from build123d import *

# Parameters (mm, degrees)
SKETCH1_W                     = 30
SKETCH1_H                     = 13.6
MAIN_SHAPE_DEPTH              = 6.35
SHOULDER_X_MOUNT_HOLES_D      = 1.9939
SHOULDER_X_MOUNT_HOLES_DEPTH  = 7.67
SHOULDER_X_MOUNT_HOLES_TIP    = 0.599027994
ELBOW_SERVO_MOUNT_HOLES_D     = 1.9939
ELBOW_SERVO_MOUNT_HOLES_DEPTH = 7.67
ELBOW_SERVO_MOUNT_HOLES_TIP   = 0.599027994
FILLET2_R                     = 3
WEIGHT_REMOVAL_DEPTH          = 7.35


with BuildPart() as part:
    # Sketch1 → main shape (new body)
    with BuildSketch(Plane.XY):
        Polygon((0, 0), (120, 0), (120, 30), (0, 30), (0, 17.159), (30, 17.159), (30, 12.841), (0, 12.841), align=None)
        with Locations((99, 15)):
            Rectangle(SKETCH1_W, SKETCH1_H, mode=Mode.SUBTRACT)
    extrude(amount=MAIN_SHAPE_DEPTH)

    # shoulder X mount holes
    with Locations(Plane.XY.offset(6.35)):
        with Locations((26.625, 26.625), (26.625, 3.375), (3.375, 3.375), (3.375, 26.625)):
            Hole(SHOULDER_X_MOUNT_HOLES_D / 2, depth=SHOULDER_X_MOUNT_HOLES_DEPTH)
            with Locations((0, 0, -(SHOULDER_X_MOUNT_HOLES_DEPTH + SHOULDER_X_MOUNT_HOLES_TIP / 2))):  # 118° drill point
                Cone(0, SHOULDER_X_MOUNT_HOLES_D / 2, SHOULDER_X_MOUNT_HOLES_TIP, mode=Mode.SUBTRACT)

    # elbow servo mount holes
    with Locations(Plane.XY.offset(6.35)):
        with Locations((81.5, 15), (116.5, 15)):
            Hole(ELBOW_SERVO_MOUNT_HOLES_D / 2, depth=ELBOW_SERVO_MOUNT_HOLES_DEPTH)
            with Locations((0, 0, -(ELBOW_SERVO_MOUNT_HOLES_DEPTH + ELBOW_SERVO_MOUNT_HOLES_TIP / 2))):  # 118° drill point
                Cone(0, ELBOW_SERVO_MOUNT_HOLES_D / 2, ELBOW_SERVO_MOUNT_HOLES_TIP, mode=Mode.SUBTRACT)

    # Fillet2
    fillet2_edges = [part.edges().sort_by_distance(p)[0] for p in [
        (0, 30, 3.175),
        (120, 30, 3.175),
        (120, 0, 3.175),
        (0, 0, 3.175),
    ]]
    fillet(fillet2_edges, radius=FILLET2_R)

    # Sketch8 → weight removal (cut, through all)
    with BuildSketch(Plane.XY):
        Polygon((36.41522176, 26), (55.5, 16.669663972), (74.58477824, 26), align=None)
        Polygon((36.41522176, 4), (74.58477824, 4), (55.5, 13.330336028), align=None)
        Polygon((78, 24.330336028), (78, 5.669663972), (58.91522176, 15), align=None)
        Polygon((33, 24.330336028), (52.08477824, 15), (33, 5.669663972), align=None)
    extrude(amount=WEIGHT_REMOVAL_DEPTH, mode=Mode.SUBTRACT)


solid = part.part
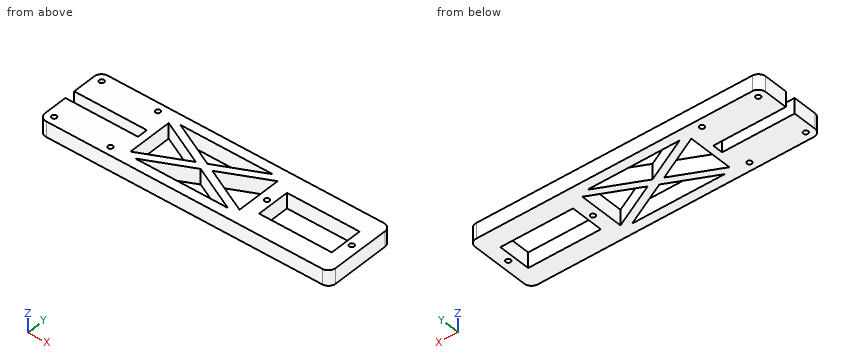
Could you check a few things on this model? Use its own coordinates, in mm. Give positions to 0.01 mm unless a question says otherwise; leave off trailing zeros. Order: outer loops, then holes, each group sorted by start corner. A loop starts at its lowest first (then second) coordinate and runs counter-clockwise, first axis right, second up. Notation, with made-up numbers: M 68.5,51 L 125.5,51 A27 ccw 125.5,87 Z; hole C 42.25,25 d10. An arc over 180 degrees is marked long. One line per question, with ' | ' between items.
1. I want a section at D-D (z = 4.5). Give the number of separate pieces and of enclosed holes in the cut face, and give its area (3 significant figures).
Results:
separate pieces: 1 | enclosed holes: 11 | area: 2,320 mm²
2. I want a section at A-A (x = 18). List the corners of the cut face in (y, z) for me, and give its area (3 significant figures).
Results:
outline: M 0,0 L 12.84,0 L 12.84,6.35 L 0,6.35 Z; M 17.16,0 L 30,0 L 30,6.35 L 17.16,6.35 Z | area: 163 mm²
3. I want a section at B-B (y = 7). List the corners of the cut face in (x, z) for me.
Results:
outline: M 0,0 L 33,0 L 33,6.35 L 0,6.35 Z; M 35.72,0 L 42.55,0 L 42.55,6.35 L 35.72,6.35 Z; M 68.45,0 L 75.28,0 L 75.28,6.35 L 68.45,6.35 Z; M 78,0 L 120,0 L 120,6.35 L 78,6.35 Z
4. I want a section at C-C (x = 54.5). List the corners of the cut face in (y, z) for me, and give its area (3 significant figures).
Results:
outline: M 0,0 L 4,0 L 4,6.35 L 0,6.35 Z; M 12.84,0 L 17.16,0 L 17.16,6.35 L 12.84,6.35 Z; M 26,0 L 30,0 L 30,6.35 L 26,6.35 Z | area: 78.2 mm²
5. I'm going to push a flat-ended pin straight in: pin 1 (1.2 mm diameter, centred on x = 3.375, y = 26.625, fed in from -Z). Where does the tip first touch, or does it pass through?
Results:
pin 1: through
6. If I drill on line 1 (Y direction, x = 90, z = 2.25); line 2 (X direction, y = 19.75, z = 2.75); line 3 (X direction, y = 19, z = 5), over which ranges is the centre line in solid material (lowest first)?
Results:
line 1: 0 to 8.2, 21.8 to 30 | line 2: 0 to 33, 42.37 to 49.2, 61.8 to 68.63, 78 to 84, 114 to 120 | line 3: 0 to 33, 43.9 to 50.73, 60.27 to 67.1, 78 to 84, 114 to 120
